The model under review builds one solid part; all positions refer to its coordinate system, in mm. Face numbers are marked on the shaded views. Give positions to 0.01 mm unless a question says otherwise; leave off trailing zeros. Loops run counter-clockwise (first coordinate to the right, second up) from the corner with the lowest first, then second, coordinate; pieces in that order, holes last. Notation, with made-up numbers: M 83,-33.75 L 110,-33.75 A21 ccw 110,0.25 Z; hole C 45,13 d1. An arc over 180 degrees is marked long. One line per item, written item: value. Start each with the question number.
Q1. We need section B-B on x = 0. Write out the cut boundary in (y, z), plus the area to 3 significant figures.
Q2. We need section C-C on x = -42.5. Write out the cut boundary in (y, z).
Q3. We need section A-A on y = 0. Write out the cut boundary in (x, z), plus the area to 4 significant figures.
Q4. For pin 1 (5.5 mm diameter, centred on x = -18.5, y = 6, fed in from +Z); pin 2 (4 mm diameter, centred on x = 18.5, y = -6, fed in from -Z); pin 3 (4 mm diameter, centred on x = -28, y = -5, fed in from +Z); pin 4 (0.8 mm diameter, centred on y = 5, z = 4.5, fed in from -X), all flat-tipped, find the tip position at first contact; note any pin that passes through.
Q5. Mouldability with a two-part tool opening along X and no side actions: class the marked faces 1 and 2 as released by +X, released by -X, zero draft, split by the parting line, or undercut.
Q6. To check wall thickness, follow line 1 along Y through (x, z) = (-18.5, 3.3); line 2 along X through (y, z) = (0.5, 3.65); line 3 along X through (y, z) = (2.75, 0.35). State the ranges of each line that lie inside material, in increasing order. Write a range as from..to.
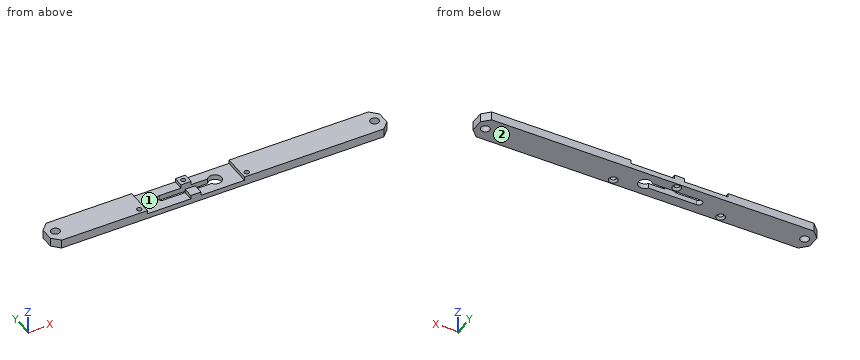
```python
from build123d import *

# Parameters (mm, degrees)
SKETCH_1_W                   = 232
SKETCH_1_H                   = 19
EXTRUDE_1_DEPTH              = 6
SKETCH_3_W                   = 30
SKETCH_3_H                   = 19
CUT_EXTRUDE_2_DEPTH          = 2.5
SKETCH_5_R                   = 3
CUT_EXTRUDE_4_DEPTH          = 117.542910552
SKETCH_4_R                   = 4.5
CUT_EXTRUDE_3_DEPTH          = 117.542910552
CHAMFER_1_SIZE               = 5
HOLE_WIZARD_M6_1_D           = 3.3
HOLE_WIZARD_M6_1_CSINK_D     = 6
HOLE_WIZARD_M6_1_CSINK_ANGLE = 90


with BuildPart() as part:
    # 草图1 → 凸台-拉伸1 (new body)
    with BuildSketch(Plane.XY):
        Rectangle(SKETCH_1_W, SKETCH_1_H)
    extrude(amount=EXTRUDE_1_DEPTH)

    # 草图3 → 切除-拉伸2 (cut)
    with BuildSketch(Plane.XY.offset(6)):
        with Locations((-37, 0)):
            Rectangle(SKETCH_3_W, SKETCH_3_H)
        Rectangle(SKETCH_3_W, SKETCH_3_H)
    extrude(amount=-CUT_EXTRUDE_2_DEPTH, mode=Mode.SUBTRACT)

    # 草图5 → 切除-拉伸4 (cut, through all)
    with BuildSketch(Plane.XY.offset(6)):
        with Locations((110, 0)):
            Circle(SKETCH_5_R)
        with Locations((-110, 0)):
            Circle(SKETCH_5_R)
    extrude(amount=-CUT_EXTRUDE_4_DEPTH, mode=Mode.SUBTRACT)

    # 草图4 → 切除-拉伸3 (cut, through all)
    with BuildSketch(Plane.XY.offset(6)):
        Circle(SKETCH_4_R)
        with BuildLine():
            Line((-37, 2.5), (0, 2.5))
            ThreePointArc((0, 2.5), (2.5, 0), (0, -2.5))
            Line((0, -2.5), (-37, -2.5))
            ThreePointArc((-37, -2.5), (-39.5, 0), (-37, 2.5))
        make_face()
    extrude(amount=-CUT_EXTRUDE_3_DEPTH, mode=Mode.SUBTRACT)

    # 倒角1
    chamfer_1_edges = [part.edges().sort_by_distance(p)[0] for p in [
        (-116, 9.5, 3),
        (116, 9.5, 3),
        (116, -9.5, 3),
        (-116, -9.5, 3),
    ]]
    chamfer(chamfer_1_edges, length=CHAMFER_1_SIZE)

    # M6 内六角花形半沉头螺钉的锥形沉头孔1 (through all)
    with Locations(Plane(origin=(0, 0, 0), x_dir=(1, 0, 0), z_dir=(0, 0, -1))):
        with Locations((-18.5, -6), (-55.5, 6), (18.5, 6)):
            CounterSinkHole(HOLE_WIZARD_M6_1_D / 2, HOLE_WIZARD_M6_1_CSINK_D / 2, counter_sink_angle=HOLE_WIZARD_M6_1_CSINK_ANGLE)


solid = part.part
```
Solved:
1. outline: M -9.5,0 L -4.5,0 L -4.5,3.5 L -9.5,3.5 Z; M 4.5,0 L 9.5,0 L 9.5,3.5 L 4.5,3.5 Z
1. area: 35.0 mm2
2. outline: M -9.5,0 L 9.5,0 L 9.5,3.5 L -9.5,3.5 Z
3. outline: M -116,0 L -113,0 L -113,6 L -116,6 Z; M -107,0 L -39.5,0 L -39.5,3.5 L -52,3.5 L -52,6 L -107,6 Z; M 4.5,0 L 107,0 L 107,6 L 15,6 L 15,3.5 L 4.5,3.5 Z; M 113,0 L 116,0 L 116,6 L 113,6 Z
3. area: 998.5 mm2
4. pin 1: z = 6
4. pin 2: z = 1
4. pin 3: z = 3.5
4. pin 4: x = -115.9
5. face 1: undercut
5. face 2: zero draft
6. line 1: -9.5..-2.5, 2.5..4.35, 7.65..9.5
6. line 2: -116..-112.96, -107.04..-52, 15..107.04, 112.96..116
6. line 3: -116..-111.2, -108.8..-3.56, 3.56..108.8, 111.2..116
